Verification items for the finished model (mm, model axes). A direction names the side the tool comes from. Coordinates: 2 decimals unless noted, no trailing zeros. Order: outer loops, then holes, each group sorted by start corner. A loop starts at its lowest first (then second) coordinate and runs counter-clockwise, first axis right, second up. Notation, with made-up numbers: M 74.25,28 L 84.25,28 A20 cw 84.25,35 Z; hole C 86.5,-19.75 d2. An arc over 180 degrees is marked long. Return JSON: item names as keys, results as strings.
```python
from build123d import *

# Parameters (mm, degrees)
F0_W      = 13
F0_H      = 13
F1_DEPTH  = 5
F2_W      = 3.2
F2_H      = 4
F2_W_2    = 4
F2_H_2    = 3.2
F3_DEPTH  = 3.5
F4_W      = 4
F4_H      = 1.9
F4_W_2    = 1.9
F4_H_2    = 4
F5_DEPTH  = 5
F6_W      = 6.5
F6_H      = 6.5
F7_DEPTH  = 5
F10_DEPTH = 0.4
F11_DEPTH = 0.4
F12_DEPTH = 0.4
F8_R      = 1.075
F13_DEPTH = 1.5
F9_R      = 1
F14_DEPTH = 2.4
F15_COUNT = 4
F16_R     = 1


with BuildPart() as f1:
    # F0 (on Top) → F1 (new body)
    with BuildSketch(Plane.XY):
        Rectangle(F0_W, F0_H)
    extrude(amount=F1_DEPTH)

    # F2 (on face) → F3 (cut)
    with BuildSketch(Plane.XY.offset(5)):
        with Locations((1.5, 4.5)):
            Rectangle(F2_W, F2_H)
        with Locations((-4.5, 1.5)):
            Rectangle(F2_W_2, F2_H_2)
        with Locations((-1.5, -4.5)):
            Rectangle(F2_W, F2_H)
        with Locations((4.5, -1.5)):
            Rectangle(F2_W_2, F2_H_2)
    extrude(amount=-F3_DEPTH, mode=Mode.SUBTRACT)

    # F4 (on face) → F5 (cut, through all)
    with BuildSketch(Plane.XY.offset(5)):
        with Locations((-4.5, 5.55)):
            Rectangle(F4_W, F4_H)
        with Locations((-5.55, -4.5)):
            Rectangle(F4_W_2, F4_H_2)
        with Locations((4.5, -5.55)):
            Rectangle(F4_W, F4_H)
        with Locations((5.55, 4.5)):
            Rectangle(F4_W_2, F4_H_2)
    extrude(amount=-F5_DEPTH, mode=Mode.SUBTRACT)

    # F6 (on Top) → F7 (intersect, through all)
    with BuildSketch(Plane.XY):
        with Locations((-3.25, 3.25)):
            Rectangle(F6_W, F6_H)
    extrude(amount=F7_DEPTH, mode=Mode.INTERSECT)

    # F10 (add): a face of the model
    f10_faces = [f1.faces().sort_by_distance(p)[0] for p in [
        (-2.164416476, 3.3918764302, 5),
    ]]
    extrude(f10_faces, amount=F10_DEPTH)

    # F11 (add): a face of the model
    f11_faces = [f1.faces().sort_by_distance(p)[0] for p in [
        (-6.5, 2.3, 0.0709365914),
    ]]
    extrude(f11_faces, amount=F11_DEPTH)

    # F12 (add): a face of the model
    f12_faces = [f1.faces().sort_by_distance(p)[0] for p in [
        (-1.2856979405, 6.5, 2.6776887872),
    ]]
    extrude(f12_faces, amount=F12_DEPTH)

    # F8 (on face) → F13 (cut, through all)
    with BuildSketch(Plane(origin=(0, 4.6, 0), x_dir=(-1, 0, 0), z_dir=(0, 1, 0))):
        with Locations((5, 3.5)):
            Circle(F8_R)
    extrude(amount=-F13_DEPTH, mode=Mode.SUBTRACT)

    # F9 (on face) → F14 (cut, through all)
    with BuildSketch(Plane.YZ.offset(-0.1)):
        with Locations((5, 3.5)):
            Circle(F9_R)
    extrude(amount=-F14_DEPTH, mode=Mode.SUBTRACT)

    # F15: F1 ×4 about axis
    f15_axis = Axis((0, 0, 2.5), (0, 0, 1))


with BuildPart() as f1_1:
    add(f1.part)
    for i in range(1, F15_COUNT):
        add(f1.part.rotate(f15_axis, i * 360 / F15_COUNT))

    # F16
    f16_edges = [f1_1.edges().sort_by_distance(p)[0] for p in [
        (6.9, 1.3, 5.4),
        (-6.9, 3.85, 5.4),
        (-1.3, 6.9, 5.4),
        (-3.85, -6.9, 5.4),
        (-6.9, -1.3, 5.4),
        (6.9, -3.85, 5.4),
        (1.3, -6.9, 5.4),
        (3.85, 6.9, 5.4),
    ]]
    fillet(f16_edges, radius=F16_R)


solid = f1_1.part
```
Q1. Tool access check on faces 4 (the face through (4.6, 5, 2)), 5 (the face through (-5, 4.6, 2)), 6 (the face through (3.7, 0.1, 3.5)), 7 (the face through (-3.7, -0.1, 3.5)), 8 (the face through (-3.1, -3.7, 3.5)). Record the directions out of +Z, -Z, +X, -X, +Y, -Y that give a thin tool (end or side, any length) a straight path to the whole face; none if there is none.
Values:
{"face 4": "+Z, -Z, +X, +Y", "face 5": "+Z, -Z, -X, +Y", "face 6": "+Z, +X", "face 7": "+Z, -X", "face 8": "+Z, -Y"}
Q2. Cross-section at D-D, the plane z = 0.8. Record the boundary of the cut face in (x, y).
Values:
{"outline": "M -6.9,-2.5 L -4.6,-2.5 L -4.6,-6.9 L 2.5,-6.9 L 2.5,-4.6 L 6.9,-4.6 L 6.9,2.5 L 4.6,2.5 L 4.6,6.9 L -2.5,6.9 L -2.5,4.6 L -6.9,4.6 Z"}
Q3. Material ranges on line 1 along Y through (x, z) = (-6, 2.25); line 2 along Z through (x, y) = (-1.65, 5), recorded low to high.
Values:
{"line 1": "-2.5 to -0.1, 3.1 to 4.6", "line 2": "0 to 2.5, 4.5 to 5.4"}
Q4. Cross-section at A-A, the plane y = -0.5. Record the boundary of the cut face in (x, z), and give its area (3 significant figures).
Values:
{"outline": "M -6.9,0 L 6.9,0 L 6.9,1.5 L 2.5,1.5 L 2.5,5.4 L -5.9,5.4 A1 ccw -6.9,4.4 Z; hole C -5,3.5 d2", "area": "54.0 mm^2"}
Q5. Draft check along Z on faces 1 (the face through (3.7, -3.1, 3.5)), 2 (the face through (-1, -5, 1.5)), 3 (the face through (4.87, 1.28, 4.49)). Enter one of: pulls with the +Z half, pulls with the -Z half, needs draft (parallel to the pull), parting line crosses it, or undercut.
Values:
{"face 1": "needs draft", "face 2": "pulls with the +Z half", "face 3": "undercut"}
Q6. Cross-section at B-B, the plane x = -5. Record the boundary of the cut face in (y, z) (3 decimals).
Values:
{"outline": "M -2.5,0 L 4.6,0 L 4.6,2.425 L 3.1,2.425 L 3.1,1.5 L -0.1,1.5 L -0.1,2.5 L -2.5,2.5 Z; M -2.5,4.5 L -0.1,4.5 L -0.1,5.4 L -2.5,5.4 Z; M 3.1,4.575 L 4.6,4.575 L 4.6,5.4 L 3.1,5.4 Z"}
Q7. Go/stop test with flat-tipped pins: pin 1 (1.2 mm diameter, centred on x = -6, z = 1.5, fed in from -Y); pin 2 (1.2 mm diameter, centred on x = 5, z = 3.5, fed in from -Y); pin 3 (3 mm diameter, centred on x = 3, z = 4, fed in from +Y); pin 4 (1.3 mm diameter, centred on y = -5.5, z = 3, fed in from -X). Record where each tip stops, or that it passes through.
Values:
{"pin 1": "y = -2.5", "pin 2": "y = 2.5", "pin 3": "y = 6.9", "pin 4": "x = -4.6"}
Q8. Cross-section at C-C, the plane y = -5. Record the boundary of the cut face in (x, z) (3 decimals), and give its area (3 significant figures).
Values:
{"outline": "M -4.6,0 L 2.5,0 L 2.5,2.5 L 0.1,2.5 L 0.1,1.5 L -3.1,1.5 L -3.1,2.425 L -4.6,2.425 Z; M -4.6,4.575 L -3.1,4.575 L -3.1,5.4 L -4.6,5.4 Z; M 0.1,4.5 L 2.5,4.5 L 2.5,5.4 L 0.1,5.4 Z", "area": "17.8 mm^2"}
